from build123d import *

# Parameters (mm, degrees)
BOSS_EXTRUDE1_DEPTH = 10
SKETCH2_R           = 1.55
CUT_EXTRUDE1_DEPTH  = 10
SKETCH3_R           = 1.55
CUT_EXTRUDE2_DEPTH  = 10
FILLET1_R           = 3
FILLET2_R           = 3
FILLET3_R           = 1


with BuildPart() as part:
    # Sketch1 → Boss-Extrude1 (new body)
    with BuildSketch(Plane.XY):
        Polygon((6.1, 10.1), (-6.1, 10.1), (-6.1, 0), (-18.1, 0), (-18.1, 2), (-8.1, 2), (-8.1, 12.1), (8.1, 12.1), (8.1, 2), (18.1, 2), (18.1, 0), (6.1, 0), align=None)
    extrude(amount=BOSS_EXTRUDE1_DEPTH)

    # Sketch2 → Cut-Extrude1 (cut)
    with BuildSketch(Plane(origin=(0, 2, 0), x_dir=(1, 0, 0), z_dir=(0, 1, 0))):
        with Locations((-13.1, -5)):
            Circle(SKETCH2_R)
    extrude(amount=-CUT_EXTRUDE1_DEPTH, mode=Mode.SUBTRACT)

    # Sketch3 → Cut-Extrude2 (cut)
    with BuildSketch(Plane(origin=(0, 2, 0), x_dir=(1, 0, 0), z_dir=(0, 1, 0))):
        with Locations((13.1, -5)):
            Circle(SKETCH3_R)
    extrude(amount=-CUT_EXTRUDE2_DEPTH, mode=Mode.SUBTRACT)

    # Fillet1
    fillet1_edges = [part.edges().sort_by_distance(p)[0] for p in [
        (-18.1, 1, 0),
        (18.1, 1, 0),
    ]]
    fillet(fillet1_edges, radius=FILLET1_R)

    # Fillet2
    fillet2_edges = [part.edges().sort_by_distance(p)[0] for p in [
        (-8.1, 12.1, 5),
        (8.1, 12.1, 5),
    ]]
    fillet(fillet2_edges, radius=FILLET2_R)

    # Fillet3
    fillet3_edges = [part.edges().sort_by_distance(p)[0] for p in [
        (6.1, 10.1, 5),
        (-6.1, 10.1, 5),
    ]]
    fillet(fillet3_edges, radius=FILLET3_R)


solid = part.part
CAD build for the part. Positions are in the model's coordinates, mm. A direction names the side the tool comes from. Coordinates: 2 decimals unless noted, no trailing zeros. Loops run counter-clockwise (first coordinate to the right, second up) from the corner with the lowest first, then second, coordinate; pieces in that order, holes last. Notation, with made-up numbers: (25, 24) -> (48, 24) arc R13 ccw to (48, 44) -> close; hole circle Ø1 at (31, 24). An arc over 180 degrees is marked (long way). One line per item, written item: value.
1. Slice it at B-B on y = 5. Write the cut outline in (x, z), and give its area (3 significant figures).
Answers:
outline: (-8.1, 0) -> (-6.1, 0) -> (-6.1, 10) -> (-8.1, 10) -> close; (6.1, 0) -> (8.1, 0) -> (8.1, 10) -> (6.1, 10) -> close
area: 40.0 mm^2
2. Which spindle directions (+Z, -Z, +X, -X, +Y, -Y) get a long thin tool onto all of the face, cutting with end or side? Do faces 4 (the face through (-18.1, 1, 6)), 5 (the face through (-5.815, 9.799, 5.07)), 6 (the face through (-11, 2, 5)), 7 (the face through (8.1, 6, 5)). Say none if no direction does.
Answers:
face 4: +Z, -Z, -X, +Y, -Y
face 5: +Z, -Z, -Y
face 6: +Z, -Z, -X, +Y
face 7: +Z, -Z, +X, +Y
3. Slice it at C-C on z = 5. Write the cut outline in (x, y).
Answers:
outline: (-18.1, 0) -> (-14.65, 0) -> (-14.65, 2) -> (-18.1, 2) -> close; (-11.55, 0) -> (-6.1, 0) -> (-6.1, 9.1) arc R1 cw to (-5.1, 10.1) -> (5.1, 10.1) arc R1 cw to (6.1, 9.1) -> (6.1, 0) -> (11.55, 0) -> (11.55, 2) -> (8.1, 2) -> (8.1, 9.1) arc R3 ccw to (5.1, 12.1) -> (-5.1, 12.1) arc R3 ccw to (-8.1, 9.1) -> (-8.1, 2) -> (-11.55, 2) -> close; (14.65, 0) -> (18.1, 0) -> (18.1, 2) -> (14.65, 2) -> close
4. Slice it at A-A on x = -13.1. Write the cut outline in (y, z), and give its area (3 significant figures).
Answers:
outline: (0, 0) -> (2, 0) -> (2, 3.45) -> (0, 3.45) -> close; (0, 6.55) -> (2, 6.55) -> (2, 10) -> (0, 10) -> close
area: 13.8 mm^2
5. Pull direction X, two halves, no side cores. Call faces 1 (the face through (-8.1, 6, 5)), 2 (the face through (6.1, 4, 5)), 3 (the face through (17.2, 0.99, 0.86)): pulls with the +X half, pulls with the -X half, needs draft (parallel to the pull), parting line crosses it, or undercut.
Answers:
face 1: pulls with the -X half
face 2: undercut
face 3: pulls with the +X half
6. Drill centre lines: line 1 (X direction, y = 1.2, z = 5); line 2 (Z direction, x = -13.1, y = 1.05); line 3 (X direction, y = 7, z = 5). Where is each one in solid material? Low to high. Write a range as [from, to].
Answers:
line 1: x = [-18.1, -14.65], [-11.55, -6.1], [6.1, 11.55], [14.65, 18.1]
line 2: z = [0, 3.45], [6.55, 10]
line 3: x = [-8.1, -6.1], [6.1, 8.1]
7. Flat gauge pins, fed straight in: P1, Ø3, axis at x = -2, z = 7.5, coming from the -Y side; P2, Ø3.5, axis at y = 5.5, z = 5, coming from the -X side; P3, Ø5, axis at x = 15, z = 7, coming from the +Y side. Where does each tip first touch, or does it go through?
Answers:
P1: stops at y = 10.1
P2: stops at x = -8.1
P3: stops at y = 2
8. Slice it at D-D on z = 9. Write the cut outline in (x, y).
Answers:
outline: (-18.1, 0) -> (-6.1, 0) -> (-6.1, 9.1) arc R1 cw to (-5.1, 10.1) -> (5.1, 10.1) arc R1 cw to (6.1, 9.1) -> (6.1, 0) -> (18.1, 0) -> (18.1, 2) -> (8.1, 2) -> (8.1, 9.1) arc R3 ccw to (5.1, 12.1) -> (-5.1, 12.1) arc R3 ccw to (-8.1, 9.1) -> (-8.1, 2) -> (-18.1, 2) -> close
